Source: three-view drawing plus pictorial views. Frame: mm from the lowest corner of the part. A direction names the side the tool comes from. Round coordinates to 2 decimals unless told otherwise and drop trailing zeros. Order: outer loops, then holes, each group sorted by start corner. A loop starts at its lowest first (then second) coordinate and runs counter-clockwise, first axis right, second up. Notation, with made-up numbers: M -3.75,-7.5 L 3.25,-7.5 A24 cw 3.25,31.5 Z; hole C 69,87 d11. An arc over 180 degrees is marked long. Return JSON: item names as keys, results as strings. Group by question number.
Q1. Contact query for flat-ended pins moving along their axis: pin 1 (5 mm diameter, centred on x = 48.5, y = 314, fed in from -Z); pin 2 (1.5 mm diameter, centred on y = 105, z = 109, fed in from +X); pin 3 (4 mm diameter, centred on x = 165, y = 89, fed in from +Z). Output: stop coordinate, or through.
Q2. Cut plane B-B on z = 80. Output: boundary loops of the cut face in (x, y), and give its area (3 significant figures).
Q3. Cut plane D-D on x = 122.5. Output: boundary loops of the cut face in (y, z).
Q4. Ray query, probe 1 along Y at (x, z) = (128, 74); probe 2 along Y at (x, z) = (130.5, 104); probe 3 along Z at (x, y) = (141, 326). Return the intervals inside material, ascending.
Q5. Cut plane C-C on z = 133. Output: boundary loops of the cut face in (x, y), and give its area (3 significant figures).
Q6. Mould query, pull axis Y, two halves, no side actions, for the marked faces 1, 2 and 3. Classes: released by +Y, released by -Y, zero draft, split by the parting line, or undercut.
Q7. Cut plane A-A on y = 50. Output: boundary loops of the cut face in (x, z), and give its area (3 significant figures).
Q8. Access query for the marked faces 4, 5 and 6. Directions: +Z, -Z, +X, -X, +Y, -Y. A direction counts if a zero-diameter tool reaches every point of the face in a straight line with its end or side. Return the directions, or none.
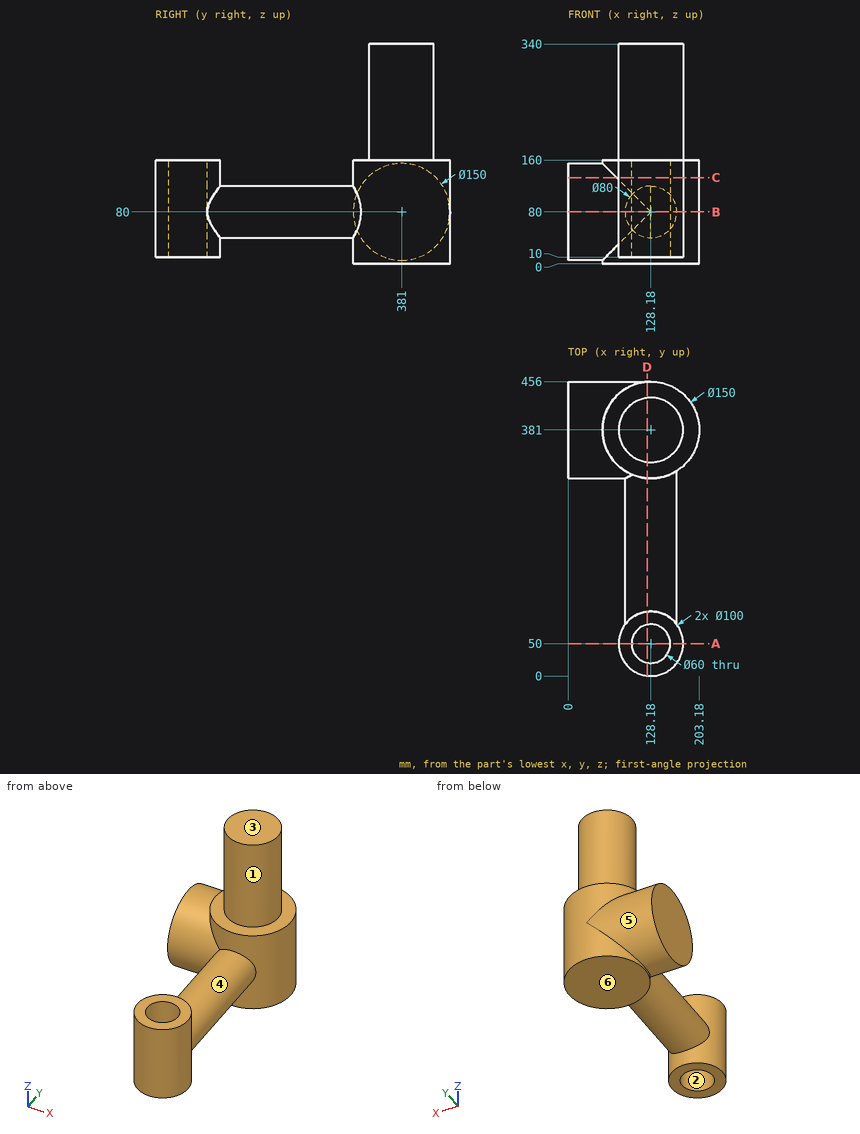
Result sheet:
{
 "1": {"pin 1": "stops at z = 41.73", "pin 2": "stops at x = 156.5", "pin 3": "stops at z = 99.69"},
 "2": {"outline": "M 0,306 L 88.18,306 L 88.18,80 A50 ccw long 168.18,80 L 168.18,317.56 A75 ccw 128.18,456 L 0,456 Z; hole C 128.18,50 d60", "area": "50,200 mm²"},
 "3": {"outline": "M 0.32,10 L 20.54,10 L 20.54,160 L 0.32,160 Z; M 79.46,10 L 99.68,10 L 99.68,40.41 L 306.22,40.41 L 306.22,0 L 455.78,0 L 455.78,74.32 A75 ccw 455.78,85.68 L 455.78,160 L 430.68,160 L 430.68,340 L 331.32,340 L 331.32,160 L 306.22,160 L 306.22,119.59 L 99.68,119.59 L 99.68,160 L 79.46,160 Z"},
 "4": {"probe 1": "y = 0 to 20, 80 to 456", "probe 2": "y = 0.05 to 20.09, 79.91 to 455.96", "probe 3": "z = 0 to 160"},
 "5": {"outline": "M 0,327.93 L 75.18,327.93 A75 ccw long 75.18,434.07 L 0,434.07 Z; C 128.18,50 d100; hole C 128.18,50 d60", "area": "29,100 mm²"},
 "6": {"face 1": "split by the parting line", "face 2": "undercut", "face 3": "zero draft"},
 "7": {"outline": "M 78.18,10 L 98.18,10 L 98.18,160 L 78.18,160 Z; M 158.18,10 L 178.18,10 L 178.18,160 L 158.18,160 Z", "area": "6,000 mm²"},
 "8": {"face 4": "none", "face 5": "-X", "face 6": "-Z, +X, -X, +Y, -Y"}
}
